Geometry check sheet. Reference: the model listing, model coordinates, mm. Face numbers are marked on the shaded views. A direction names the side the tool comes from. Round coordinates to 2 decimals unless told otherwise and drop trailing zeros. Order: outer loops, then holes, each group sorted by start corner. A loop starts at its lowest first (then second) coordinate and runs counter-clockwise, first axis right, second up.
(1) Set-up check for the marked faces 1 and 2: record each of +Z, -Z, +X, -X, +Y, -Y from which the full face is reachable in a straight line by a thin tool's end or side.
(2) Sectioned sample at C-C (x = 3.5). Record the boundary of the cut face in (y, z).
(3) Go/stop test with flat-tipped pins: pin 1 (2.5 mm diameter, centred on x = -14.76, y = -15.4, fed in from -Z); pin 2 (0.9 mm diameter, centred on y = 1, z = 3, fed in from +X); pin 3 (1 mm diameter, centred on x = -6, z = 2, fed in from +Y). Record where each tip stops, or that it passes through.
(4) Sectioned sample at A-A (x = 15.5). Record the boundary of the cut face in (y, z).
(5) Sectioned sample at D-D (z = 2.2). Record the boundary of the cut face in (x, y), plus the area to 3 significant figures.
(6) Sectioned sample at B-B (y = 0). Record the boundary of the cut face in (x, z).
(7) Material ranges on line 1 along X through (y, z) = (-9.5, 3); line 2 along Y through (x, z) = (6, 1.95); line 3 along Z through (x, y) = (-12.5, 2), recorded low to high.
from build123d import *

# Parameters (mm, degrees)
F0_W     = 35
F0_H     = 35
F1_DEPTH = 1
F3_D     = 3
F4_W     = 24.421909
F4_H     = 24.421909
F5_DEPTH = 3


with BuildPart() as f1:
    # F0 (on Top) → F1 (new body)
    with BuildSketch(Plane.XY):
        with Locations((0.242682, -0.403982)):
            Rectangle(F0_W, F0_H)
    extrude(amount=F1_DEPTH)

    # F3 (through all)
    with Locations(Plane.XY.offset(1)):
        with Locations((-14.757318, 14.596018), (-14.757318, -15.403982), (15.242682, -15.403982), (15.242682, 14.596018)):
            Hole(F3_D / 2)

    # F4 (on face) → F5 (join)
    with BuildSketch(Plane.XY.offset(1)):
        with Locations((0.242682, -0.403982)):
            Rectangle(F4_W, F4_H)
    extrude(amount=F5_DEPTH)


solid = f1.part
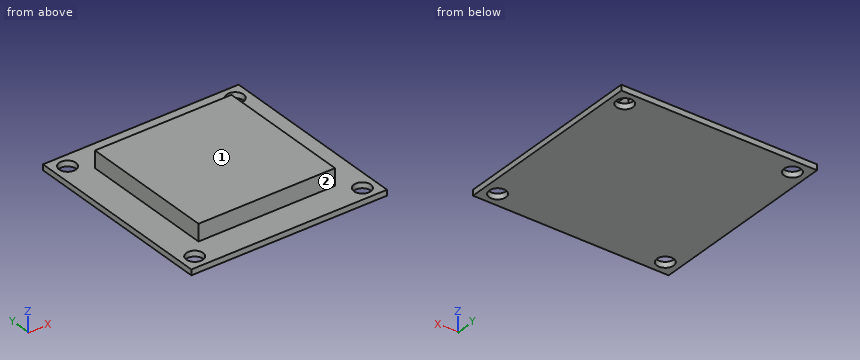
Answer below:
1. face 1: +Z, +X, -X, +Y, -Y
1. face 2: +Z, +X, -X, -Y
2. outline: (-17.9, 0) - (17.1, 0) - (17.1, 1) - (11.81, 1) - (11.81, 4) - (-12.61, 4) - (-12.61, 1) - (-17.9, 1) - close
3. pin 1: passes through
3. pin 2: stops at x = 12.45
3. pin 3: stops at y = 11.81
4. outline: (-17.9, 0) - (-16.88, 0) - (-16.88, 1) - (-17.9, 1) - close; (-13.93, 0) - (13.12, 0) - (13.12, 1) - (-13.93, 1) - close; (16.07, 0) - (17.1, 0) - (17.1, 1) - (16.07, 1) - close
5. outline: (-11.97, -12.61) - (12.45, -12.61) - (12.45, 11.81) - (-11.97, 11.81) - close
5. area: 596 mm2
6. outline: (-17.26, 0) - (17.74, 0) - (17.74, 1) - (12.45, 1) - (12.45, 4) - (-11.97, 4) - (-11.97, 1) - (-17.26, 1) - close
7. line 1: x = -11.97 to 12.45
7. line 2: y = -12.61 to 11.81
7. line 3: z = 0 to 1
